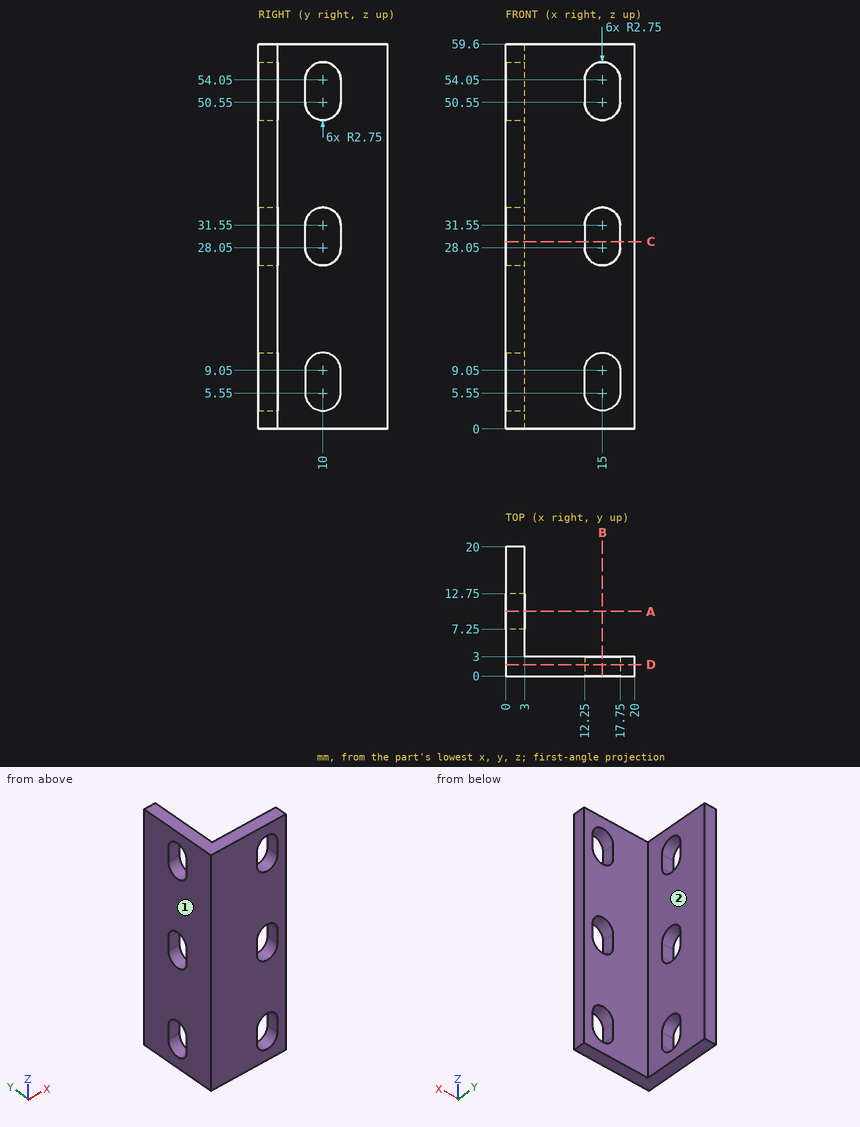
Input: dimensioned drawing with shaded views. Units: mm. Origin: part minimum x, y, z. A direction names the side the tool comes from. Give positions to 0.01 mm unless a question says otherwise; leave off trailing zeros. Write each loop counter-clockwise with the first axis right and the second up, starting at its lowest first coordinate (ties: lowest second). Pieces come first, ordered by that corner, then holes. Notation, with made-up numbers: (-5.75, 8) - (29.25, 8) arc R25 ccw to (29.25, 44) - close; hole circle Ø5 at (-9, 73.5). An arc over 180 degrees is marked (long way). Write item = value, one per line. Start each with the question number.
1) Cut plane D-D (y = 1.75). Return loops of the section in (x, z), and give its area (3 significant figures).
2) Cut plane C-C (z = 29). Return loops of the section in (x, y).
3) Cut plane A-A (y = 10). Return loops of the section in (x, z).
4) Pin query (flat end, axial travel): pin 1 (8.5 mm diameter, centred on x = 12.5, z = 17, fed in from +Y); pin 2 (3 mm diameter, centred on y = 13, z = 39.5, fed in from +X). Return the tip coordinate at first contact, or that it passes through.
5) Reachability of the marked faces 1 and 2 from +Z, -Z, +X, -X, +Y, -Y: full face, straight path, thin tool, end or side. Return the list, or none.
6) Material intervals for L1, parallel to Z at x = 2.5, y = 10.25; L2, parallel to X at y = 2, z = 50.5; L3, parallel to X at y = 16.5, z = 26, sorted ascending. Write a range as [from, to].
Answers follow:
q1.outline = (0, 0) - (20, 0) - (20, 59.6) - (0, 59.6) - close; hole (12.25, 5.55) arc R2.75 ccw to (17.75, 5.55) - (17.75, 9.05) arc R2.75 ccw to (12.25, 9.05) - close; hole (12.25, 28.05) arc R2.75 ccw to (17.75, 28.05) - (17.75, 31.55) arc R2.75 ccw to (12.25, 31.55) - close; hole (12.25, 50.55) arc R2.75 ccw to (17.75, 50.55) - (17.75, 54.05) arc R2.75 ccw to (12.25, 54.05) - close
q1.area = 1,060 mm^2
q2.outline = (0, 0) - (12.25, 0) - (12.25, 3) - (3, 3) - (3, 7.25) - (0, 7.25) - close; (0, 12.75) - (3, 12.75) - (3, 20) - (0, 20) - close; (17.75, 0) - (20, 0) - (20, 3) - (17.75, 3) - close
q3.outline = (0, 0) - (3, 0) - (3, 2.8) - (0, 2.8) - close; (0, 11.8) - (3, 11.8) - (3, 25.3) - (0, 25.3) - close; (0, 34.3) - (3, 34.3) - (3, 47.8) - (0, 47.8) - close; (0, 56.8) - (3, 56.8) - (3, 59.6) - (0, 59.6) - close
q4.pin_1 = 3
q4.pin_2 = 3
q5.face_1 = +Z, -Z, -X, +Y, -Y
q5.face_2 = +Z, -Z, +X, +Y
q6.L1 = [0, 2.81], [11.79, 25.31], [34.29, 47.81], [56.79, 59.6]
q6.L2 = [0, 12.25], [17.75, 20]
q6.L3 = [0, 3]
